Source: three-view drawing plus pictorial views. Frame: mm from the lowest corner of the part. Give positions to 0.01 mm unless a question says otherwise; leave off trailing zeros. Order: outer loops, then holes, each group sorted by start corner. A loop starts at its lowest first (then second) coordinate and runs counter-clockwise, first axis right, second up. Notation, with made-up numbers: (49, 79.25) -> (57, 79.25) arc R9 cw to (57, 91.25) -> close; hole circle Ø10 at (13.25, 42). An arc over 180 degrees is marked (long way). Answer in a Markdown table with one row per item.
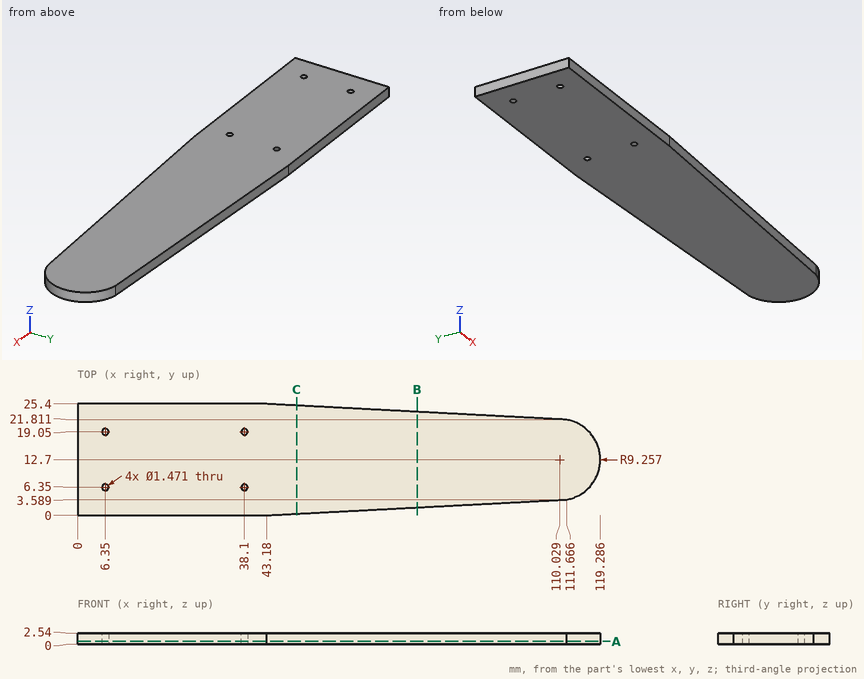
(1) Section query B-B (x = 77.5). Return the cut outline in (y, z).
A:
| item | result |
|---|---|
| outline | (1.8, 0) -> (23.6, 0) -> (23.6, 2.54) -> (1.8, 2.54) -> close |
(2) Ray query, probe 1 along Y at (x, z) = (6.35, 1.45) (1 decimal); probe 2 along X at (y, z) = (12.25, 0.4) (1 decimal); probe 3 along X at (y, z) = (5, 2.25) (1 decimal). Return the intervals inside material, ascending.
A:
| item | result |
|---|---|
| probe 1 | y = 0 to 5.6, 7.1 to 18.3, 19.8 to 25.4 |
| probe 2 | x = 0 to 119.3 |
| probe 3 | x = 0 to 115.2 |
(3) Section query A-A (z = 0.7). Give the number of separate pieces and of enclosed holes in the cut face, plus the area to 3 significant figures.
A:
| item | result |
|---|---|
| separate pieces | 1 |
| enclosed holes | 4 |
| area | 2,690 mm^2 |
(4) First-contact query: pin 1 Ø1.3 at (x, y) = (6.35, 19.05) entering from +Z; pin 2 Ø1 at (y, z) = (12, 2) entering from +X. Flat tips, straight axial feed; report the tip coordinate or a pass-through.
A:
| item | result |
|---|---|
| pin 1 | passes through |
| pin 2 | stops at x = 119.28 |
(5) Section query C-C (x = 50). Return the cut outline in (y, z), plus the area to 3 significant figures.
A:
| item | result |
|---|---|
| outline | (0.36, 0) -> (25.04, 0) -> (25.04, 2.54) -> (0.36, 2.54) -> close |
| area | 62.7 mm^2 |
